Could you check a few things on this model? Use its own coordinates, in mm. A direction names the side the tool comes from. Round coordinates to 2 decimals unless told otherwise and drop trailing zeros. Order: outer loops, then holes, each group sorted by start corner. A loop starts at its lowest first (then second) coordinate and runs counter-clockwise, first axis right, second up. Notation, with made-up numbers: (-18.5, 10.25) - (-2.5, 10.25) arc R22 ccw to (-2.5, 20.25) - close; hole circle Ø9 at (54, 46.5). An arc over 180 degrees is marked (long way). Use one line per item in the form item = value.
from build123d import *

# Parameters (mm, degrees)
F1_DEPTH    = 10
F2_T1_DEPTH = 34.4948974279
F2_T3_DEPTH = 35
F3_R        = 1
F4_R        = 1.75
F5_DEPTH    = 20.001
F6_SIZE     = 2


# Not quite as in the source:
# - a fillet or chamfer that OpenCascade refuses, or shapes differently, is made with other operations: its cross-section is extruded or revolved along the edge and cut away or added


with BuildPart() as f1:
    # F0 (on Front) → F1 (new body)
    with BuildSketch(Plane.XZ):
        Polygon((-18.6188016892, 16), (-18.6188016892, 20), (-36.6188016892, 20), (-36.6188016892, 0), (-18.6188016892, 0), (-18.6188016892, 10), (-22.6188016892, 10), (-22.6188016892, 4), (-32.6188016892, 4), (-32.6188016892, 16), align=None)
    extrude(amount=F1_DEPTH)

    # F2: fillet of radius 5 on 3 edges, made by hand

    # F2_s2 → F2_t1 (cut)
    with BuildSketch(Plane.XZ.offset(-12.2474487139)):
        with BuildLine():
            ThreePointArc((-23.5177811747, 16), (-20.3555035146, 17.1270166538), (-18.6188016892, 20))
            Line((-18.6188016892, 20), (-18.6188016892, 16))
            Line((-18.6188016892, 16), (-23.5177811747, 16))
        make_face()
    extrude(amount=F2_T1_DEPTH, mode=Mode.SUBTRACT)

    # F2_s4 → F2_t3 (cut)
    with BuildSketch(Plane.XZ.offset(-12.5)):
        with BuildLine():
            ThreePointArc((-18.6188016892, 5), (-20.0832677832, 1.4644660941), (-23.6188016892, 0))
            Line((-23.6188016892, 0), (-18.6188016892, 0))
            Line((-18.6188016892, 0), (-18.6188016892, 5))
        make_face()
        with BuildLine():
            ThreePointArc((-36.6188016892, 5), (-35.1543355951, 1.4644660941), (-31.6188016892, 0))
            Line((-31.6188016892, 0), (-36.6188016892, 0))
            Line((-36.6188016892, 0), (-36.6188016892, 5))
        make_face()
    extrude(amount=F2_T3_DEPTH, mode=Mode.SUBTRACT)

    # F3
    f3_edges = [f1.edges().sort_by_distance(p)[0] for p in [
        (-18.618802, -5, 10),
        (-22.618802, -5, 10),
        (-32.618802, -5, 16),
    ]]
    fillet(f3_edges, radius=F3_R)

    # F4 (on face) → F5 (cut, through all)
    with BuildSketch(Plane.XY.offset(20)):
        with Locations((-27.6188016892, -5)):
            Circle(F4_R)
    extrude(amount=-F5_DEPTH, mode=Mode.SUBTRACT)

    # F6
    f6_edges = [f1.edges().sort_by_distance(p)[0] for p in [
        (-29.368802, -5, 16),
    ]]
    chamfer(f6_edges, length=F6_SIZE)


solid = f1.part
Item 1: Imagine slicing it at B-B on z = 4.25. Please give me the cut outline in (x, y).
Found:
outline = (-36.56, -10) - (-32.62, -10) - (-32.62, 0) - (-36.56, 0) - close; (-22.62, -10) - (-18.68, -10) - (-18.68, 0) - (-22.62, 0) - close
Item 2: Imagine slicing it at A-A on y = -5. Please give me the cut outline in (x, z), plus the area to 3 significant figures.
Found:
outline = (-36.62, 5) arc R5 ccw to (-31.62, 0) - (-29.37, 0) - (-29.37, 4) - (-32.62, 4) - (-32.62, 15) arc R1 cw to (-31.62, 16) - (-31.37, 16) - (-29.37, 18) - (-29.37, 20) - (-36.62, 20) - close; (-25.87, 0) - (-23.62, 0) arc R5 ccw to (-18.62, 5) - (-18.62, 9) arc R1 ccw to (-19.62, 10) - (-21.62, 10) arc R1 ccw to (-22.62, 9) - (-22.62, 4) - (-25.87, 4) - close; (-25.87, 18) - (-23.87, 16) - (-23.52, 16) arc R5 ccw to (-18.62, 20) - (-25.87, 20) - close
area = 168 mm2
Item 3: I need wall thicknesses on L1, parallel to Z at x = -28.25, y = -9; L2, parallel to X at y = -0.75, z = 5; L3, parallel to X at y = -9.5, z = 10.75. Which ranges of each line are inside material? Lowest first, please.
Found:
L1 = 0 to 4, 16 to 20
L2 = -36.62 to -32.62, -22.62 to -18.62
L3 = -36.62 to -32.62
Item 4: Imagine slicing it at D-D on x = -27.5. State how many separate pieces and enclosed holes the cut face has, plus the area to 3 significant figures.
Found:
separate_pieces = 4
enclosed_holes = 0
area = 48.1 mm2
Item 5: If we mould it in two halves opening along Y, with no side actions, what happens to faces 4 (the face through (-34, -10, 10)), 5 (the face through (-26, -5.67, 2.03)), 6 (the face through (-20.045, -4.93, 1.504)), 7 (the face through (-34, 0, 10))? For each: released by +Y, released by -Y, zero draft, split by the parting line, or undercut.
Found:
face_4 = released by -Y
face_5 = undercut
face_6 = zero draft
face_7 = released by +Y
Item 6: Imagine slicing it at C-C on x = -20.75. Please give me the cut outline in (y, z), plus the area to 3 significant figures.
Found:
outline = (-10, 0.9) - (0, 0.9) - (0, 10) - (-10, 10) - close; (-10, 16.84) - (0, 16.84) - (0, 20) - (-10, 20) - close
area = 123 mm2
Item 7: For faces 1 (the face through (-22.334, -5.07, 9.699)), 2 (the face through (-18.619, -5, 7)), 3 (the face through (-32.318, -5.07, 15.715)), which set-ups out of +Z, -Z, +X, -X, +Y, -Y let a thin tool reach every point of the face, with its end or its side?
Found:
face_1 = +Y, -Y
face_2 = +Z, -Z, +X, +Y, -Y
face_3 = +X, +Y, -Y
